Model file for the job. Use its own axes, mm. A direction names the side the tool comes from. Give positions to 0.01 mm unless a question says otherwise; leave off trailing zeros. Loops run counter-clockwise (first coordinate to the right, second up) from the corner with the lowest first, then second, coordinate; pieces in that order, holes last. Notation, with made-up numbers: M 22,-34 L 63,-34 A15 cw 63,-13 Z; hole C 36.25,53 d4. An arc over 180 degrees is marked long. Use CSV: the item, a comma, the result in double quotes. Start each with the question number.
(1) Slice it at B-B on z = 0. List the corners of the cut face in (x, y), and give its area (4 significant figures).
(2) Flat gauge pins, fed straight in: P1, Ø2, axis at y = 2.5, z = -2.5, coming from the -X side; P2, Ø2, axis at x = 1, z = 0.5, coming from the +Y side; P3, Ø2, axis at x = 0, z = 0, coming from the +Y side. Where does each tip first touch, or does it go through?
(3) Two-plate mould, pull along X, no slides. Class faces 1 (the face through (-2.3, 3.5, 0.7)), 2 (the face through (1, 1, -1)), 3 (the face through (-3.417, 1.726, -0.759)): pulls with the +X half, pulls with the -X half, needs draft (parallel to the pull), parting line crosses it, or undercut.
(4) Slice it at C-C on y = 1.9. List the corners of the cut face in (x, z), and give its area (3 significant figures).
(5) Wall check: line 1 along X through (y, z) = (2.85, 0); line 2 along X through (y, z) = (1.7, 0); line 3 along Z through (x, y) = (1, 2.45). Give the ranges that are in metal, low to high. Write a range as from..to.
(6) Slice it at D-D on z = 1.5. List the corners of the cut face in (x, y), and give its area (3 significant figures).
(7) Tool access for faces 4 (the face through (-1, 2, 1)), 5 (the face through (-2, 0, 2)), 6 (the face through (-1.952, 0.493, 0.434)): list every direction of +Z, -Z, +X, -X, +Y, -Y with a clear straight run to the whole face (end or side of a thin tool).
(8) Slice it at A-A on x = 0. List the corners of the cut face in (y, z).
```python
from build123d import *

# Parameters (mm, degrees)
SKETCH1_R           = 3.5
BOSS_EXTRUDE1_DEPTH = 2
SKETCH2_R           = 3.5
SKETCH2_R_2         = 2.25
BOSS_EXTRUDE2_DEPTH = 1.5
SKETCH3_R           = 2
CUT_EXTRUDE1_DEPTH  = 1
SKETCH4_R           = 1.25
CUT_EXTRUDE2_DEPTH  = 1


with BuildPart() as part:
    # Sketch1 → Boss-Extrude1 (new body)
    with BuildSketch(Plane(origin=(0, 0, 0), x_dir=(1, 0, 0), z_dir=(0, 1, 0))):
        with Locations(Location((0, 0, 0), (0, 0, 270))):
            Circle(SKETCH1_R)
    extrude(amount=BOSS_EXTRUDE1_DEPTH)

    # Sketch2 → Boss-Extrude2 (add)
    with BuildSketch(Plane(origin=(0, 2, 0), x_dir=(1, 0, 0), z_dir=(0, 1, 0))):
        with Locations(Location((0, 0, 0), (0, 0, 270))):
            Circle(SKETCH2_R)
        with Locations(Location((0, 0, 0), (0, 0, 270))):
            Circle(SKETCH2_R_2, mode=Mode.SUBTRACT)
    extrude(amount=BOSS_EXTRUDE2_DEPTH)

    # Sketch3 → Cut-Extrude1 (cut)
    with BuildSketch(Plane.XZ):
        with Locations(Location((0, 0, 0), (0, 0, 270))):
            Circle(SKETCH3_R)
    extrude(amount=-CUT_EXTRUDE1_DEPTH, mode=Mode.SUBTRACT)

    # Sketch4 → Cut-Extrude2 (cut)
    with BuildSketch(Plane.XZ.offset(-1)):
        with Locations(Location((0, 0, 0), (0, 0, 270))):
            Circle(SKETCH4_R)
    extrude(amount=-CUT_EXTRUDE2_DEPTH, mode=Mode.SUBTRACT)


solid = part.part
```
Reply:
1,outline,"M -3.5,0 L -2,0 L -2,1 L -1.25,1 L -1.25,2 L -2.25,2 L -2.25,3.5 L -3.5,3.5 Z; M 1.25,1 L 2,1 L 2,0 L 3.5,0 L 3.5,3.5 L 2.25,3.5 L 2.25,2 L 1.25,2 Z"
1,area,"11.25 mm^2"
2,P1,"stops at x = -3.16"
2,P2,"stops at y = 2"
2,P3,"passes through"
3,face 1,"needs draft"
3,face 2,"undercut"
3,face 3,"parting line crosses it"
4,outline,"C 0,0 d7; hole C 0,0 d2.5"
4,area,"33.6 mm^2"
5,line 1,"x = -3.5..-2.25, 2.25..3.5"
5,line 2,"x = -3.5..-1.25, 1.25..3.5"
5,line 3,"z = -3.35..-2.02, 2.02..3.35"
6,outline,"M -3.16,0 L -1.32,0 L -1.32,1 L 1.32,1 L 1.32,0 L 3.16,0 L 3.16,3.5 L 1.68,3.5 L 1.68,2 L -1.68,2 L -1.68,3.5 L -3.16,3.5 Z"
6,area,"14.5 mm^2"
7,face 4,"+Y"
7,face 5,"+Z, -Z, +X, -X, -Y"
7,face 6,"-Y"
8,outline,"M 0,-3.5 L 3.5,-3.5 L 3.5,-2.25 L 2,-2.25 L 2,-1.25 L 1,-1.25 L 1,-2 L 0,-2 Z; M 0,2 L 1,2 L 1,1.25 L 2,1.25 L 2,2.25 L 3.5,2.25 L 3.5,3.5 L 0,3.5 Z"
